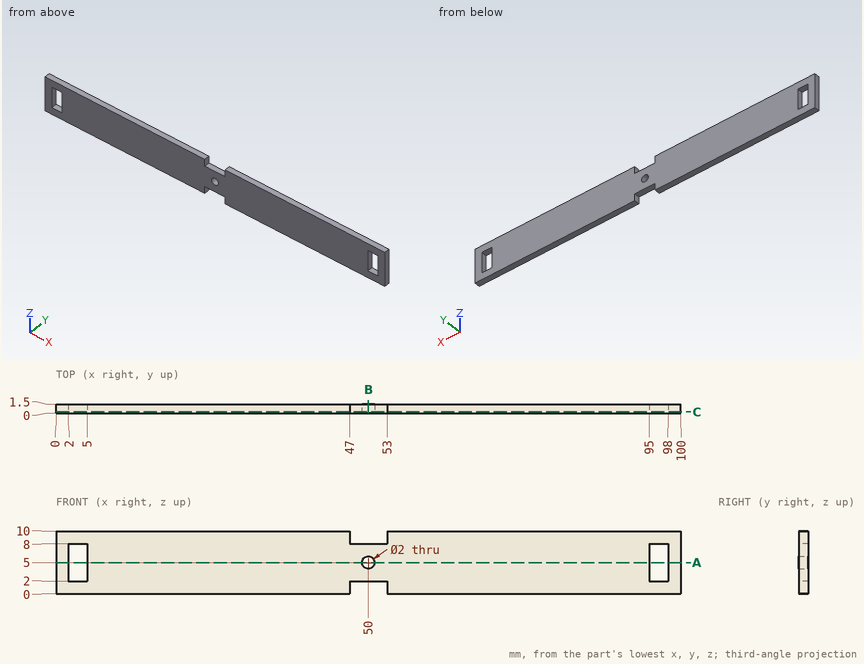
Study the drawing (mm; zero at the part's minimum x, y, z) and answer. Give positions to 0.01 mm unless a question says otherwise; leave off trailing zeros. Write each loop counter-clockwise with the first axis right and the second up, starting at its lowest first coordinate (ties: lowest second). Pieces come first, ordered by that corner, then holes. Notation, with made-up numbers: M 69,22 L 84,22 A33 cw 84,53 Z; hole C -32,86.5 d5. An arc over 180 degrees is marked long. Put each result on its own line as item: value. Start each with the question number.
1. The part is cut by section C-C, the plane y = 0.25. Give the vertices of the cut face in (x, z), and give its area (3 significant figures).
2. Consider line 1 along X through (y, z) = (0.65, 5); line 2 along X through (y, z) = (0.35, 3.5); line 3 along X through (y, z) = (0.5, 8.25). Determine where each line is inside the solid, lowest interval first.
3. The part is cut by section A-A, the plane z = 5. Give the vertices of the cut face in (x, y).
4. The part is cut by section B-B, the plane x = 50. Give the vertices of the cut face in (y, z), and give its area (3 significant figures).
Final values:
1. outline: M 0,0 L 47,0 L 47,2 L 53,2 L 53,0 L 100,0 L 100,10 L 53,10 L 53,8 L 47,8 L 47,10 L 0,10 Z; hole M 2,2 L 5,2 L 5,8 L 2,8 Z; hole C 50,5 d2; hole M 95,2 L 98,2 L 98,8 L 95,8 Z
1. area: 937 mm²
2. line 1: x = 0 to 2, 5 to 49, 51 to 95, 98 to 100
2. line 2: x = 0 to 2, 5 to 95, 98 to 100
2. line 3: x = 0 to 47, 53 to 100
3. outline: M 0,0 L 2,0 L 2,1.5 L 0,1.5 Z; M 5,0 L 49,0 L 49,1.5 L 5,1.5 Z; M 51,0 L 95,0 L 95,1.5 L 51,1.5 Z; M 98,0 L 100,0 L 100,1.5 L 98,1.5 Z
4. outline: M 0,2 L 1.5,2 L 1.5,4 L 0,4 Z; M 0,6 L 1.5,6 L 1.5,8 L 0,8 Z
4. area: 6.00 mm²
